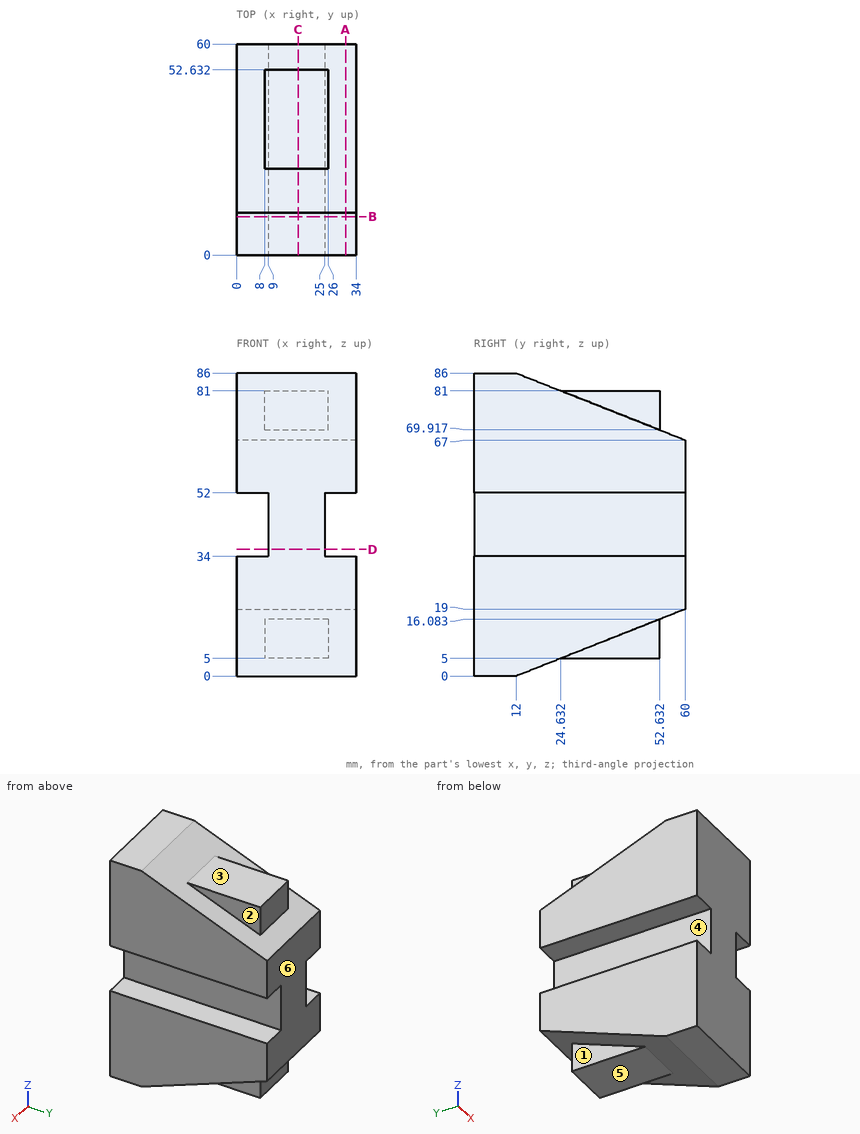
Design review of the part shown in the three views and the two pictorial views. Dimensions are in mm from the part's minimum x, y and z. A direction names the side the tool comes from. Round coordinates to 2 decimals unless told otherwise and drop trailing zeros. Loops run counter-clockwise (first coordinate to the right, second up) from the corner with the lowest first, then second, coordinate; pieces in that order, holes last. Notation, with made-up numbers: (89.5, 13.5) - (129.5, 13.5) arc R6 ccw to (129.5, 19.5) - close; hole circle Ø1 at (-5, 35.25). An arc over 180 degrees is marked (long way). Use CSV: the item, a comma, the result in double quotes.
(1) Machinability: for the marked faces 1, 2 and 3, which of the approach directions +Z, -Z, +X, -X, +Y, -Y give a long, thin tool a straight path to every point of the face, cutting with its end or side? Answer none if there is none.
Working result:
face 1,"-Z, -X, +Y"
face 2,"+Z, +X, +Y"
face 3,"+Z, +X, -X, +Y"
(2) Take a section at D-D, the plane z = 36. Give the boundary of the cut face in (x, y).
Working result:
outline,"(9, 0) - (25, 0) - (25, 60) - (9, 60) - close"
(3) Take a section at B-B, the plane y = 11. Give the boundary of the cut face in (x, z), plus the area to 3 significant figures.
Working result:
outline,"(0, 0) - (34, 0) - (34, 34) - (25, 34) - (25, 52) - (34, 52) - (34, 86) - (0, 86) - (0, 52) - (9, 52) - (9, 34) - (0, 34) - close"
area,"2,600 mm^2"
(4) Take a section at A-A, the plane x = 31. Give the boundary of the cut face in (y, z).
Working result:
outline,"(0, 0) - (12, 0) - (60, 19) - (60, 34) - (0, 34) - close; (0, 52) - (60, 52) - (60, 67) - (12, 86) - (0, 86) - close"
(5) The part is to be moulded in two halves that separate along Z. For the marked faces 4, 5 and 6, say which applies: pulls with the +Z half, pulls with the -Z half, needs draft (parallel to the pull), parting line crosses it, or undercut.
Working result:
face 4,"undercut"
face 5,"pulls with the -Z half"
face 6,"needs draft"
(6) Take a section at C-C, the plane x = 17.5. Give the boundary of the cut face in (y, z), plus the area to 3 significant figures.
Working result:
outline,"(0, 0) - (12, 0) - (24.63, 5) - (52.63, 5) - (52.63, 16.08) - (60, 19) - (60, 67) - (52.63, 69.92) - (52.63, 81) - (24.63, 81) - (12, 86) - (0, 86) - close"
area,"4,560 mm^2"
(7) For line 1 (Z direction, x = 29.5, y = 10.5); line 2 (Z direction, x = 24.5, y = 41); line 3 (Z direction, x = 27, y = 28), list the stretches that pass through material, from the lowest coordinate up.
Working result:
line 1,"z = 0 to 34, 52 to 86"
line 2,"z = 5 to 81"
line 3,"z = 6.33 to 34, 52 to 79.67"
(8) Clearance check with flat-ended pins moving along their axes: P1, Ø2.5, axis at x = 30.5, y = 25, coming from the -Z side; P2, Ø5, axis at y = 33.5, z = 41, coming from the -X side; P3, Ø7, axis at x = 6.5, y = 17.5, coming from the -Z side. State where each tip first meets the part, or that it passes through.
Working result:
P1,"stops at z = 4.65"
P2,"stops at x = 9"
P3,"stops at z = 0.79"
